The model under review builds one solid part; all positions refer to its coordinate system, in mm. Face numbers are marked on the shaded views. Round coordinates to 2 decimals unless told otherwise and drop trailing zeros. Order: outer loops, then holes, each group sorted by start corner. A loop starts at its lowest first (then second) coordinate and runs counter-clockwise, first axis right, second up. Notation, with made-up numbers: M 5.5,56 L 18.5,56 A11 ccw 18.5,69 Z; hole C -0.75,62 d4. An arc over 180 degrees is marked long. Use a Markdown table: item, result. Add a question column.
1. Consider section C-C on x = -1.5. State the section outline as (y, z) points, then the cut area to 3 significant figures.
2. Insertion check: P1, Ø5, axis at y = 0, z = 125, coming from the +X side; P2, Ø2.5, axis at y = 0, z = 60, coming from the +X side. Each pin has a flat end and moves straight along its axis. Give the tip position at first contact, or say it passes through.
3. To check wall thickness, follow probe 1 along Z at (x, y) = (6.8, 0); probe 2 along Y at (x, z) = (6.75, 125); probe 3 along X at (y, z) = (-4, 86.5). State the ranges of each line that lie inside material, in increasing order.
4. The part is to be moulded in two halves that separate along X. For the marked faces 1, 2 and 3, say which applies: +X half, -X half, draft (parallel to the pull), parting line (faces both ways), or undercut.
5. Consider section B-B on y = 0. State the section outline as (x, z) points, then the cut area to 3 significant figures.
6. Consider section A-A on z = 86. State the section outline as (x, y) points, then the cut area to 3 significant figures.
7. Consider section D-D on z = 60. State the section outline as (x, y) points, then the cut area to 3 significant figures.
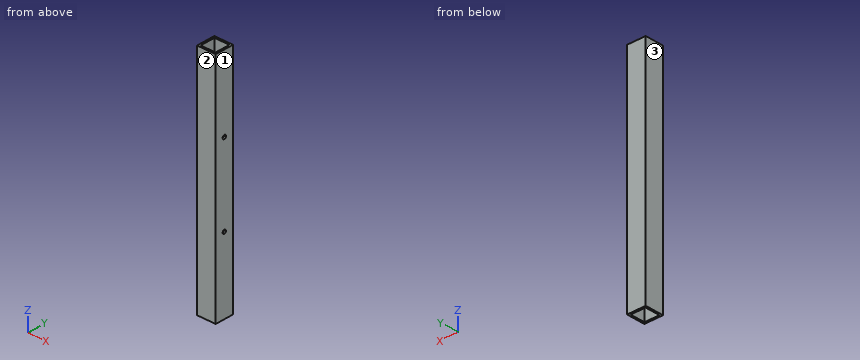
from build123d import *

# Parameters (mm, degrees)
SKETCH_W     = 15
SKETCH_H     = 15
SKETCH_W_2   = 12
SKETCH_H_2   = 12
PAD_DEPTH    = 185
SKETCH001_R  = 1.5
POCKET_DEPTH = 5


with BuildPart() as part:
    # Sketch → Pad (new body)
    with BuildSketch(Plane.XY):
        Rectangle(SKETCH_W, SKETCH_H)
        Rectangle(SKETCH_W_2, SKETCH_H_2, mode=Mode.SUBTRACT)
    extrude(amount=PAD_DEPTH)

    # Sketch001 → Pocket (cut)
    with BuildSketch(Plane.YZ.offset(7.5)):
        with Locations((0, 60)):
            Circle(SKETCH001_R)
        with Locations((0, 125)):
            Circle(SKETCH001_R)
    extrude(amount=-POCKET_DEPTH, mode=Mode.SUBTRACT)


solid = part.part
Answer block:
| question | item | result |
|---|---|---|
| 1 | outline | M -7.5,0 L -6,0 L -6,185 L -7.5,185 Z; M 6,0 L 7.5,0 L 7.5,185 L 6,185 Z |
| 1 | area | 555 mm^2 |
| 2 | P1 | x = 7.5 |
| 2 | P2 | x = -6 |
| 3 | probe 1 | 0 to 58.5, 61.5 to 123.5, 126.5 to 185 |
| 3 | probe 2 | -7.5 to -1.5, 1.5 to 7.5 |
| 3 | probe 3 | -7.5 to -6, 6 to 7.5 |
| 4 | face 1 | +X half |
| 4 | face 2 | draft |
| 4 | face 3 | -X half |
| 5 | outline | M -7.5,0 L -6,0 L -6,185 L -7.5,185 Z; M 6,0 L 7.5,0 L 7.5,58.5 L 6,58.5 Z; M 6,61.5 L 7.5,61.5 L 7.5,123.5 L 6,123.5 Z; M 6,126.5 L 7.5,126.5 L 7.5,185 L 6,185 Z |
| 5 | area | 546 mm^2 |
| 6 | outline | M -7.5,-7.5 L 7.5,-7.5 L 7.5,7.5 L -7.5,7.5 Z; hole M -6,-6 L 6,-6 L 6,6 L -6,6 Z |
| 6 | area | 81.0 mm^2 |
| 7 | outline | M -7.5,-7.5 L 7.5,-7.5 L 7.5,-1.5 L 6,-1.5 L 6,-6 L -6,-6 L -6,6 L 6,6 L 6,1.5 L 7.5,1.5 L 7.5,7.5 L -7.5,7.5 Z |
| 7 | area | 76.5 mm^2 |
